from build123d import *

# Parameters (mm, degrees)
SKETCH_1_R               = 26
EXTRUDE_1_DEPTH          = 2
CHAMFER_2_SIZE           = 0.6
PATTERN_CIRCULAR_1_COUNT = 8


with BuildPart() as part:
    # Эскиз1 → Бобышка-Вытянуть1 (new body)
    with BuildSketch(Plane.XY):
        Circle(SKETCH_1_R)
    extrude(amount=EXTRUDE_1_DEPTH)

    # Фаска2
    chamfer_2_edges = [part.edges().sort_by_distance(p)[0] for p in [
        (-26, 0, 2),
    ]]
    chamfer(chamfer_2_edges, length=CHAMFER_2_SIZE)

    # Эскиз3 → Зенковка для винта с полупотайной головкой M21 (revolve, cut)
    with BuildSketch(Plane(origin=(-23, 0, 2), x_dir=(0, -1, 0), z_dir=(1, 0, 0))):
        Polygon((0, 0), (0, 6.721032743), (1.2, 6), (1.2, 1), (2.2, 0), align=None)
    hole_wizard_m21 = revolve(axis=Axis((-23, 0, 8.35), (0, 0, -1)), mode=Mode.SUBTRACT)

    # Круговой массив1: Зенковка для винта с полупотайной головкой M21 ×8 about axis
    pattern_circular_1_axis = Axis((0, 0, 0), (0, 0, 1))
    for i in range(1, PATTERN_CIRCULAR_1_COUNT):
        add(hole_wizard_m21.rotate(pattern_circular_1_axis, i * 360 / PATTERN_CIRCULAR_1_COUNT), mode=Mode.SUBTRACT)


solid = part.part
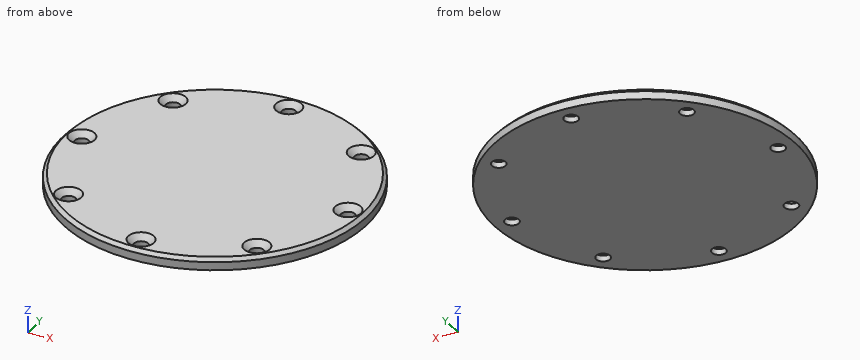
Input: part model. Units: mm. Frame: model coordinates. Give positions to 0.01 mm unless a question says otherwise; leave off trailing zeros. Loops run counter-clockwise (first coordinate to the right, second up) from the corner with the lowest first, then second, coordinate; pieces in that order, holes last. Notation, with made-up numbers: (72, 37) - (107, 37) arc R8 cw to (107, 41) - close; hole circle Ø8 at (78, -12.5). An arc over 180 degrees is marked (long way). Use CSV: the item, a comma, the result in double quotes. Start each with the question number.
Item 1: Section A-A on y = 0. Return loops of the section in (x, z), then the cut area to 3 significant figures.
Item 2: Line query: line 1 (Y direction, x = 0.5, z = 0.7); line 2 (X direction, y = 16.5, z = 0.7). Output: solid intervals per line, ascending.
Item 3: Section B-B on z = 0.4. State how many separate pieces and enclosed holes the cut face has, then the cut area to 3 significant figures.
Item 4: Contact query for flat-ended pins moving along their axis: P1, Ø1.9, axis at x = -23, y = 0, coming from the +Z side; P2, Ø3, axis at x = 16.26, y = -16.26, coming from the +Z side. Output: stop coordinate, or through.
Ans:
1,outline,"(-26, 0) - (-24.2, 0) - (-24.2, 1) - (-25.2, 2) - (-25.4, 2) - (-26, 1.4) - close; (-21.8, 0) - (21.8, 0) - (21.8, 1) - (20.8, 2) - (-20.8, 2) - (-21.8, 1) - close; (24.2, 0) - (26, 0) - (26, 1.4) - (25.4, 2) - (25.2, 2) - (24.2, 1) - close"
1,area,"92.0 mm2"
2,line 1,"y = -26 to -24.09, -21.91 to 21.91, 24.09 to 26"
2,line 2,"x = -20.09 to -17.44, -15.09 to 15.09, 17.44 to 20.09"
3,separate pieces,"1"
3,enclosed holes,"8"
3,area,"2,090 mm2"
4,P1,"passes through"
4,P2,"stops at z = 1.3"
